Geometry: final body of the model. Coordinates: model frame, mm. A direction names the side the tool comes from. Give positions to 0.01 mm unless a question says otherwise; leave off trailing zeros. Write each loop counter-clockwise with the first axis right and the second up, starting at its lowest first coordinate (ties: lowest second). Pieces come first, ordered by that corner, then holes. Notation, with made-up numbers: (39.5, -16.5) -> (46.5, -16.5) arc R17 cw to (46.5, 4.5) -> close; hole circle Ø2 at (-15, 89). An arc over 180 degrees is marked (long way). Answer in a Markdown table with one row per item. Add a question column.
Item 1: Section query A-A on z = 4.75. Output: boundary loops of the cut face in (x, y).
Item 2: Draft query along Y for faces 3 (the cylindrical face through (-0.59, 4.46, 1.43)), 4 (the flat face through (-5, 0, 4)), 5 (the flat face through (0, 3.8, 5)), 6 (the cylindrical face through (-1.4, 0.06, 3.54)). Return one class per face: +Y half, -Y half, draft (parallel to the pull), parting line (faces both ways), or undercut.
Item 3: Material intervals for probe 1 along X at (y, z) = (0, 3.95); probe 2 along Z at (x, y) = (2, 1), sorted ascending. Write a range as from..to.
Item 4: First-contact query: P1, Ø3, axis at x = 0.5, z = 2.5, coming from the -Y side; P2, Ø6, axis at x = 2, y = 0.5, coming from the +Z side. Flat tips, straight axial feed; report the tip coordinate or a pass-through.
Item 5: Access query for faces 1 (the flat face through (0, -3, 0)), 2 (the flat face through (-1.3, 1.3, 2.9)). Directions: +Z, -Z, +X, -X, +Y, -Y. A direction counts if a zero-diameter tool reaches every point of the face in a straight line with its end or side. Return the directions, or none.
```python
from build123d import *

# Parameters (mm, degrees)
ESQUISSE1_R                = 4.5
BOSS_EXTRU_1_DEPTH         = 2.9
ESQUISSE2_W                = 10
ESQUISSE2_H                = 10
ESQUISSE2_R                = 1.4
BOSS_EXTRU_2_DEPTH         = 1.3
ESQUISSE3_W                = 10
ESQUISSE3_H                = 1.2
BOSS_EXTRU_3_DEPTH         = 2
ENL_V_MAT_EXTRU_1_DEPTH    = 7.6
R_P_TITION_LIN_AIRE4_COUNT = 20
R_P_TITION_LIN_AIRE4_PITCH = 0.5


with BuildPart() as part:
    # Esquisse1 → Boss.-Extru.1 (new body)
    with BuildSketch(Plane.XY):
        Circle(ESQUISSE1_R)
        Polygon((2.011577371, -1.550856692), (2.011577371, -2.011577371), (1.550856692, -2.011577371), (1.541643286, -2.018647066), (1.4224, -2.463669069), (0.977377998, -2.344425783), (0.966648759, -2.348869979), (0.73628842, -2.747865791), (0.337292608, -2.517505451), (0.325778716, -2.519021284), (0, -2.8448), (-0.325778716, -2.519021284), (-0.337292608, -2.517505451), (-0.73628842, -2.747865791), (-0.966648759, -2.348869979), (-0.977377998, -2.344425783), (-1.4224, -2.463669069), (-1.541643286, -2.018647066), (-1.550856692, -2.011577371), (-2.011577371, -2.011577371), (-2.011577371, -1.550856692), (-2.018647066, -1.541643286), (-2.463669069, -1.4224), (-2.344425783, -0.977377998), (-2.348869979, -0.966648759), (-2.747865791, -0.73628842), (-2.517505451, -0.337292608), (-2.519021284, -0.325778716), (-2.8448, 0), (-2.519021284, 0.325778716), (-2.517505451, 0.337292608), (-2.747865791, 0.73628842), (-2.348869979, 0.966648759), (-2.344425783, 0.977377998), (-2.463669069, 1.4224), (-2.018647066, 1.541643286), (-2.011577371, 1.550856692), (-2.011577371, 2.011577371), (-1.550856692, 2.011577371), (-1.541643286, 2.018647066), (-1.4224, 2.463669069), (-0.977377998, 2.344425783), (-0.966648759, 2.348869979), (-0.73628842, 2.747865791), (-0.337292608, 2.517505451), (-0.325778716, 2.519021284), (0, 2.8448), (0.325778716, 2.519021284), (0.337292608, 2.517505451), (0.73628842, 2.747865791), (0.966648759, 2.348869979), (0.977377998, 2.344425783), (1.4224, 2.463669069), (1.541643286, 2.018647066), (1.550856692, 2.011577371), (2.011577371, 2.011577371), (2.011577371, 1.550856692), (2.018647066, 1.541643286), (2.463669069, 1.4224), (2.344425783, 0.977377998), (2.348869979, 0.966648759), (2.747865791, 0.73628842), (2.517505451, 0.337292608), (2.519021284, 0.325778716), (2.8448, 0), (2.519021284, -0.325778716), (2.517505451, -0.337292608), (2.747865791, -0.73628842), (2.348869979, -0.966648759), (2.344425783, -0.977377998), (2.463669069, -1.4224), (2.018647066, -1.541643286), align=None, mode=Mode.SUBTRACT)
    extrude(amount=BOSS_EXTRU_1_DEPTH)

    # Esquisse2 → Boss.-Extru.2 (add)
    with BuildSketch(Plane.XY.offset(2.9)):
        Rectangle(ESQUISSE2_W, ESQUISSE2_H)
        Circle(ESQUISSE2_R, mode=Mode.SUBTRACT)
    extrude(amount=BOSS_EXTRU_2_DEPTH)

    # Esquisse3 → Boss.-Extru.3 (add)
    with BuildSketch(Plane.XY.offset(4.2)):
        with Locations((0, 4.4)):
            Rectangle(ESQUISSE3_W, ESQUISSE3_H)
        with Locations((0, -4.4)):
            Rectangle(ESQUISSE3_W, ESQUISSE3_H)
    extrude(amount=BOSS_EXTRU_3_DEPTH)

    # Esquisse4 → Enlèv. mat.-Extru.1 (cut)
    with BuildSketch(Plane.XZ.offset(-3.8)):
        Polygon((-4.55, 4.2), (-4.7, 4), (-4.8, 4), (-4.95, 4.2), align=None)
    enl_v_mat_extru_1 = extrude(amount=ENL_V_MAT_EXTRU_1_DEPTH, mode=Mode.SUBTRACT)

    # Répétition linéaire4: Enlèv. mat.-Extru.1 ×20
    with Locations(*[(i * R_P_TITION_LIN_AIRE4_PITCH, 0, 0) for i in range(1, R_P_TITION_LIN_AIRE4_COUNT)]):
        add(enl_v_mat_extru_1, mode=Mode.SUBTRACT)


solid = part.part
```
Findings below:
| question | item | result |
|---|---|---|
| 1 | outline | (-5, -5) -> (5, -5) -> (5, -3.8) -> (-5, -3.8) -> close; (-5, 3.8) -> (5, 3.8) -> (5, 5) -> (-5, 5) -> close |
| 2 | face 3 | parting line |
| 2 | face 4 | draft |
| 2 | face 5 | undercut |
| 2 | face 6 | undercut |
| 3 | probe 1 | x = -5..-1.4, 1.4..5 |
| 3 | probe 2 | z = 2.9..4.2 |
| 4 | P1 | stops at y = -5 |
| 4 | P2 | stops at z = 4.2 |
| 5 | face 1 | -Z, +X, -X, +Y, -Y |
| 5 | face 2 | -Z |
